from build123d import *

# Parameters (mm, degrees)
F0_W     = 127
F0_H     = 76.2
F1_DEPTH = 25.4
F2_T     = -0.9906
F3_W     = 0.9906
F3_H     = 74.2188
F4_DEPTH = 25.4
F5_W     = 21.4376
F5_H     = 72.2376
F6_DEPTH = 25.4


with BuildPart() as f1:
    # F0 (on Front) → F1 (new body)
    with BuildSketch(Plane.XZ):
        Rectangle(F0_W, F0_H)
    extrude(amount=F1_DEPTH)

    # F2
    f2_openings = [f1.faces().sort_by_distance(p)[0] for p in [
        (0, -25.4, 0),
    ]]
    offset(amount=F2_T, openings=f2_openings)

    # F3 (on face) → F4 (join)
    with BuildSketch(Plane.XZ.offset(0.9906)):
        with Locations((54.391131, 0)):
            Rectangle(F3_W, F3_H)
    extrude(amount=F4_DEPTH)

    # F5 (on face) → F6 (cut)
    with BuildSketch(Plane(origin=(-63.5, 0, 0), x_dir=(0, -1, 0), z_dir=(-1, 0, 0))):
        with Locations((12.447563, 0.106448)):
            Rectangle(F5_W, F5_H)
    extrude(amount=-F6_DEPTH, mode=Mode.SUBTRACT)


solid = f1.part
Design review of the part built by this model. Coordinates are the model's own, in mm. A direction names the side the tool comes from. Give positions to 0.01 mm unless a question says otherwise; leave off trailing zeros. Order: outer loops, then holes, each group sorted by start corner. A loop starts at its lowest first (then second) coordinate and runs counter-clockwise, first axis right, second up. Notation, with made-up numbers: (-32.5, 42) - (6.5, 42) arc R20 cw to (6.5, 50) - close; hole circle Ø6 at (12.25, -23). An arc over 180 degrees is marked (long way). Use CSV: the item, a comma, the result in double quotes. Start each with the question number.
Q1. Take a section at A-A (z = -15.5). State the section outline as (x, y) points.
Q2. For line 1 (X direction, y = -13.25, z = -4); line 2 (Z direction, x = -46.5, y = -11); line 3 (Y direction, x = 29.5, z = -12), list the stretches that pass through material, from the lowest coordinate up.
Q3. Machinability: for faces 4 (the face through (63.5, -13, -1)), 5 (the face through (59, -13, -37.109)), which of the approach directions +Z, -Z, +X, -X, +Y, -Y give a long, thin tool a straight path to every point of the face, cutting with its end or side? Answer none if there is none.
Q4. Draft analysis for pull direction Z (two halves, no side actions). For faces 1 (the face through (-63.5, -24, -3)), 2 (the face through (-1, -13, -38.1)), 3 (the face through (59, -0.991, 1)), state which applies: pulls with the +Z half, pulls with the -Z half, needs draft (parallel to the pull), parting line crosses it, or undercut.
Q5. Take a section at B-B (y = -18.75). State the section outline as (x, z) points, and give its area (3 significant figures).
Q6. For P1, Ø1.5, axis at y = -14.5, z = -19, coming from the -X side; P2, Ø4, axis at x = 60, z = -5.5, coming from the -Y side; P3, Ø1.1, axis at x = 54, y = -26, coming from the -Z side, all flat-tipped, find the tip position at first contact; note any pin that passes through.
Q7. Take a section at C-C (x = -49). State the section outline as (y, z) points.
Calculated:
1,outline,"(-63.5, -25.4) - (-62.51, -25.4) - (-62.51, -23.17) - (-63.5, -23.17) - close; (-63.5, -1.73) - (-62.51, -1.73) - (-62.51, -0.99) - (53.9, -0.99) - (53.9, -26.39) - (54.89, -26.39) - (54.89, -0.99) - (62.51, -0.99) - (62.51, -25.4) - (63.5, -25.4) - (63.5, 0) - (-63.5, 0) - close"
2,line 1,"x = 53.9 to 54.89, 62.51 to 63.5"
2,line 2,"z = -38.1 to -37.11, 37.11 to 38.1"
2,line 3,"y = -0.99 to 0"
3,face 4,"+Z, -Z, +X, +Y, -Y"
3,face 5,"-Y"
4,face 1,"needs draft"
4,face 2,"pulls with the -Z half"
4,face 3,"undercut"
5,outline,"(-63.5, -38.1) - (63.5, -38.1) - (63.5, 38.1) - (-63.5, 38.1) - (-63.5, 36.23) - (-62.51, 36.23) - (-62.51, 37.11) - (53.9, 37.11) - (53.9, -37.11) - (-62.51, -37.11) - (-62.51, -36.01) - (-63.5, -36.01) - close; hole (54.89, -37.11) - (62.51, -37.11) - (62.51, 37.11) - (54.89, 37.11) - close"
5,area,"401 mm²"
6,P1,"stops at x = 53.9"
6,P2,"stops at y = -0.99"
6,P3,"stops at z = -37.11"
7,outline,"(-25.4, -38.1) - (0, -38.1) - (0, 38.1) - (-25.4, 38.1) - (-25.4, 37.11) - (-0.99, 37.11) - (-0.99, -37.11) - (-25.4, -37.11) - close"
